```python
from build123d import *

# Parameters (mm, degrees)
SKETCH1_R           = 10.795
SKETCH1_R_2         = 6.477
BOSS_EXTRUDE1_DEPTH = 12.7
CHAMFER1_SIZE       = 3.81


with BuildPart() as part:
    # Sketch1 → Boss-Extrude1 (new body)
    # profile 1 of 2: a face of its own
    with BuildSketch(Plane(origin=(0, 0, 0), x_dir=(1, 0, 0), z_dir=(0, 1, 0))):
        with BuildLine():
            Line((-5.01846801, 37.618275862), (-10.664244521, 1.675086207))
            ThreePointArc((-10.664244521, 1.675086207), (0, 10.795), (10.664244521, 1.675086207))
            Line((10.664244521, 1.675086207), (5.01846801, 37.618275862))
            ThreePointArc((5.01846801, 37.618275862), (0, 41.91), (-5.01846801, 37.618275862))
        make_face()
    # profile 2 of 2: a face of its own
    with BuildSketch(Plane(origin=(0, 0, 0), x_dir=(1, 0, 0), z_dir=(0, 1, 0))):
        Circle(SKETCH1_R)
        with Locations(Location((0, 0, 0), (0, 0, 270))):
            Circle(SKETCH1_R_2, mode=Mode.SUBTRACT)
    extrude(amount=BOSS_EXTRUDE1_DEPTH)

    # Chamfer1
    chamfer1_edges = [part.edges().sort_by_distance(p)[0] for p in [
        (0, 12.7, -6.477),
        (0, 0, -6.477),
    ]]
    chamfer(chamfer1_edges, length=CHAMFER1_SIZE)


solid = part.part
```
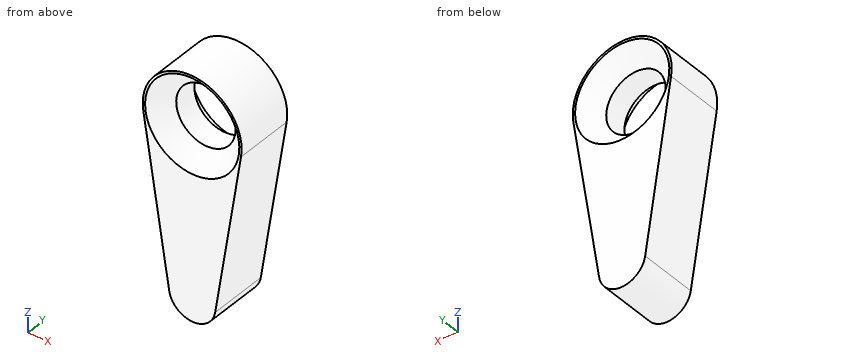
Source: CAD feature listing. Evaluate the final solid. Frame: model axes, mm. Give positions to 0.01 mm unless a question says otherwise; leave off trailing zeros. Write each loop counter-clockwise with the first axis right and the second up, starting at its lowest first coordinate (ties: lowest second). Pieces come first, ordered by that corner, then holes. Notation, with made-up numbers: (50.25, -28) - (96.25, -28) arc R32 cw to (96.25, 6) - close; hole circle Ø6 at (44.25, 78.25). An arc over 180 degrees is marked (long way). One line per item, written item: value. Start each with the question number.
Q1. Section query A-A, the plane x = 0. Return the cut outline in (y, z) (3 decimals), then the cut area to 3 significant figures.
Q2. Section query B-B, the plane z = 0. Return the cut outline in (x, y) (3 decimals), then the cut area to 3 significant figures.
Q3. First-contact query: pin 1 Ø2 at (y, z) = (1.5, 5) entering from -X; pin 2 Ø2 at (y, z) = (6, -23) entering from -X; pin 3 Ø12 at (x, z) = (-0.5, -4) entering from -Y. Flat tips, straight axial feed; report the tip coordinate or a pass-through.
Q4. Section query D-D, the plane z = -18. Return the cut outline in (x, y).
Q5. Section query C-C, the plane y = 6.25. Return the cut outline in (x, z) (3 decimals), then the cut area to 3 significant figures.
Q6. Material intervals for probe 1 along X at (y, z) = (6.35, 0) (3 decimals); probe 2 along Z at (x, y) = (-2, 9.5); probe 3 along X at (y, z) = (1.25, -6), sorted ascending. Write a range as from..to.
Answer:
1. outline: (0, -41.91) - (12.7, -41.91) - (12.7, -10.287) - (8.89, -6.477) - (3.81, -6.477) - (0, -10.287) - close; (0, 10.287) - (3.81, 6.477) - (8.89, 6.477) - (12.7, 10.287) - (12.7, 10.795) - (0, 10.795) - close
1. area: 476 mm2
2. outline: (-10.795, 0) - (-10.287, 0) - (-6.477, 3.81) - (-6.477, 8.89) - (-10.287, 12.7) - (-10.795, 12.7) - close; (6.477, 3.81) - (10.287, 0) - (10.795, 0) - (10.795, 12.7) - (10.287, 12.7) - (6.477, 8.89) - close
2. area: 80.6 mm2
3. pin 1: stops at x = -10.03
3. pin 2: stops at x = -7.47
3. pin 3: stops at y = 0.26
4. outline: (-8.1, 0) - (8.1, 0) - (8.1, 12.7) - (-8.1, 12.7) - close
5. outline: (-10.664, -1.675) - (-5.018, -37.618) arc R5.08 ccw to (5.018, -37.618) - (10.664, -1.675) arc R10.795 ccw (long way) to start; hole circle Ø12.954 at (0, 0)
5. area: 684 mm2
6. probe 1: x = -10.795..-6.477, 6.477..10.795
6. probe 2: z = -41.5..-6.8, 6.8..10.61
6. probe 3: x = -9.98..-6.76, 6.76..9.98
